Verification items for the finished model (mm, model axes). Face numbers are marked on the shaded views. Give positions to 0.01 mm unless a question says otherwise; leave off trailing zeros. Order: outer loops, then holes, each group sorted by start corner. A loop starts at its lowest first (then second) coordinate and runs counter-clockwise, first axis right, second up.
(1) Sectioned sample at A-A on y = 28.5. Count the separate pieces of the cut face and the enclosed holes in it, plus the area to 3 significant figures.
(2) Mould release check, pull along X, two halves, no side actions. Record for the marked faces 1, 2, 3 and 4: pulls with the +X half, pulls with the -X half, needs draft (parallel to the pull), parting line crosses it, or undercut.
(3) Scan lines: L1, parallel to X at y = 11.75, z = 31.75 (1 decimal); L2, parallel to X at y = 21, z = 7 (3 decimals); L3, parallel to Z at x = 62, y = 4.5. Record each from-to range of solid material in increasing order.
(4) Gauge pin test, flat ends, axial feed: pin 1 (6.5 mm diameter, centred on x = -91, z = 31, fed in from +Y); pin 2 (2 mm diameter, centred on x = 105, z = 55, fed in from +Y); pin 3 (3 mm diameter, centred on x = 64, z = 34, fed in from +Y). Record the tip position at first contact, or that the pin passes through.
(5) Sectioned sample at C-C on z = 17.5. Record the cut outline in (x, y) (3 decimals), plus the area to 3 significant figures.
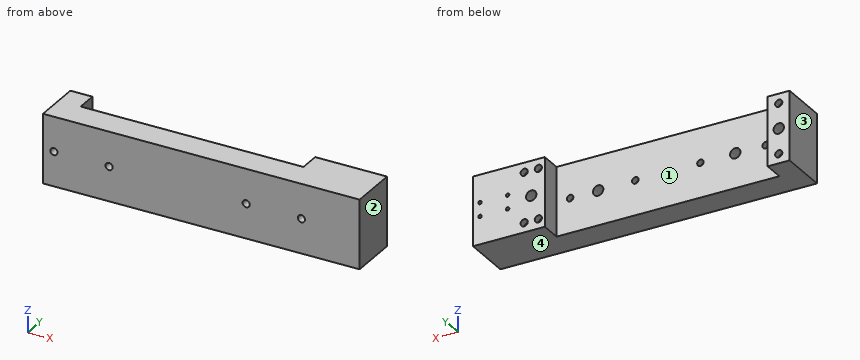
```python
from build123d import *

# Parameters (mm, degrees)
SKETCH1_W                       = 41.1
SKETCH1_H                       = 38.05
MAIN_EXTRUDE_DEPTH              = 63.5
SKETCH3_R                       = 3.3
RAIL_BLOCK_MOUNTING_HOLES_DEPTH = 6.35
SKETCH4_R                       = 1.5875
MOTOR_MOUNTING_HOLES_DEPTH      = 6.35
SKETCH8_R                       = 3
RAIL_MOUNTING_HOLES_DEPTH       = 6.35
SKETCH5_R                       = 3.31216
CUT_EXTRUDE3_DEPTH              = 39.05
CUT_EXTRUDE3_DEPTH_BACK         = 7.35
SKETCH7_R                       = 4.7625
CUT_EXTRUDE6_DEPTH              = 32.7


with BuildPart() as part:
    # Sketch1 → Main Extrude (new body)
    with BuildSketch(Plane.XY):
        Polygon((125.125, 0), (-125.125, 0), (-125.125, -6.35), (166.225, -6.35), (166.225, 0), align=None)
        Polygon((-125.125, 38.05), (-125.125, 0), (125.125, 0), (125.125, 38.05), (100.125, 38.05), (100.125, 19.05), (-104.875, 19.05), (-104.875, 38.05), align=None)
        with Locations((145.675, 19.025)):
            Rectangle(SKETCH1_W, SKETCH1_H)
    extrude(amount=MAIN_EXTRUDE_DEPTH)

    # Sketch3 → Rail Block Mounting Holes (cut)
    with BuildSketch(Plane(origin=(0, 38.05, 0), x_dir=(1, 0, 0), z_dir=(0, 1, 0))):
        with Locations((106.125, -54.75)):
            Circle(SKETCH3_R)
        with Locations((119.125, -54.75)):
            Circle(SKETCH3_R)
        with Locations((106.125, -8.75)):
            Circle(SKETCH3_R)
        with Locations((119.125, -8.75)):
            Circle(SKETCH3_R)
        with Locations((-115.125, -54.75)):
            Circle(SKETCH3_R)
        with Locations((-115.125, -8.75)):
            Circle(SKETCH3_R)
    extrude(amount=-RAIL_BLOCK_MOUNTING_HOLES_DEPTH, mode=Mode.SUBTRACT)

    # Sketch4 → Motor Mounting Holes (cut)
    with BuildSketch(Plane(origin=(0, 38.05, 0), x_dir=(1, 0, 0), z_dir=(0, 1, 0))):
        with Locations((134.373571068, -25.432199749)):
            Circle(SKETCH4_R)
        with Locations((159.773570419, -25.426458163)):
            Circle(SKETCH4_R)
        with Locations((159.77642991, -38.07645784)):
            Circle(SKETCH4_R)
        with Locations((134.376430559, -38.082199426)):
            Circle(SKETCH4_R)
    extrude(amount=-MOTOR_MOUNTING_HOLES_DEPTH, mode=Mode.SUBTRACT)

    # Sketch8 → Rail Mounting Holes (cut)
    with BuildSketch(Plane(origin=(0, 19.05, 0), x_dir=(1, 0, 0), z_dir=(0, 1, 0))):
        with Locations((87.625, -31.75)):
            Circle(SKETCH8_R)
        with Locations((27.625, -31.75)):
            Circle(SKETCH8_R)
        with Locations((-32.319, -31.75)):
            Circle(SKETCH8_R)
        with Locations((-92.263, -31.75)):
            Circle(SKETCH8_R)
    extrude(amount=-RAIL_MOUNTING_HOLES_DEPTH, mode=Mode.SUBTRACT)

    # Sketch5 → Cut-Extrude3 (cut, two sides)
    with BuildSketch(Plane(origin=(0, 0, 0), x_dir=(1, 0, 0), z_dir=(0, 1, 0))) as cut_extrude3_sk:
        with Locations((-115.125, -31.75)):
            Circle(SKETCH5_R)
        with Locations((-64.325, -31.75)):
            Circle(SKETCH5_R)
        with Locations((61.825, -31.75)):
            Circle(SKETCH5_R)
        with Locations((112.625, -31.75)):
            Circle(SKETCH5_R)
    extrude(amount=CUT_EXTRUDE3_DEPTH, mode=Mode.SUBTRACT)
    extrude(cut_extrude3_sk.sketch, amount=-CUT_EXTRUDE3_DEPTH_BACK, mode=Mode.SUBTRACT)

    # Sketch7 → Cut-Extrude6 (cut, through all)
    with BuildSketch(Plane(origin=(0, 6.35, 0), x_dir=(-1, 0, 0), z_dir=(0, -1, 0))):
        with Locations((115.125, -31.75)):
            Circle(SKETCH7_R)
        with Locations((64.325, -31.75)):
            Circle(SKETCH7_R)
        with Locations((-112.625, -31.75)):
            Circle(SKETCH7_R)
        with Locations((-61.825, -31.75)):
            Circle(SKETCH7_R)
    extrude(amount=-CUT_EXTRUDE6_DEPTH, mode=Mode.SUBTRACT)


solid = part.part
```
Ans:
1. separate pieces: 2
1. enclosed holes: 2
1. area: 5,340 mm2
2. face 1: undercut
2. face 2: pulls with the +X half
2. face 3: pulls with the -X half
2. face 4: needs draft
3. L1: x = -125.1 to -119.9, -110.4 to -69.1, -59.6 to 57.1, 66.6 to 107.9, 117.4 to 166.2
3. L2: x = -125.125 to -104.875, 100.125 to 166.225
3. L3: z = 0 to 28.44, 35.06 to 63.5
4. pin 1: stops at y = 19.05
4. pin 2: stops at y = 31.7
4. pin 3: stops at y = 6.35
5. outline: (-125.125, -6.35) - (166.225, -6.35) - (166.225, 38.05) - (100.125, 38.05) - (100.125, 19.05) - (-104.875, 19.05) - (-104.875, 38.05) - (-125.125, 38.05) - close
5. area: 9,040 mm2
